Read the model definition and answer for the solid it produces. Units are mm, in the model's axes. Round coordinates to 2 decimals unless told otherwise and drop trailing zeros. Loops run counter-clockwise (first coordinate to the right, second up) from the corner with the lowest first, then second, coordinate; pieces in that order, holes last. Notation, with made-up numbers: M 61.5,75 L 69.5,75 A21 cw 69.5,108 Z; hole C 55,34 d4. An arc over 180 degrees is marked long. Write each question's results on one line, items separated by ' | '.
```python
from build123d import *

# Parameters (mm, degrees)
CYLINDER001_R     = 1.65
CYLINDER001_DEPTH = 3
CYLINDER_R        = 3.5
CYLINDER_DEPTH    = 3
CHAMFER001_SIZE   = 0.4


with BuildPart() as cylinder001:
    # Cylinder001 → Cylinder001 (new body)
    with BuildSketch(Plane.XY):
        Circle(CYLINDER001_R)
    extrude(amount=CYLINDER001_DEPTH)


with BuildPart() as chamfer001:
    # Cylinder → Cylinder (new body)
    with BuildSketch(Plane.XY):
        Circle(CYLINDER_R)
    extrude(amount=CYLINDER_DEPTH)

    # Cut: cut Cylinder001
    add(cylinder001.part, mode=Mode.SUBTRACT)

    # Chamfer001
    chamfer001_edges = [chamfer001.edges().sort_by_distance(p)[0] for p in [
        (-3.5, 0, 0),
        (-1.65, 0, 0),
    ]]
    chamfer(chamfer001_edges, length=CHAMFER001_SIZE)


solid = chamfer001.part
```
1. Find section C-C, the plane z = 1.3. Give the vertices of the cut face in (x, y).
Completed:
outline: C 0,0 d7; hole C 0,0 d3.3
2. Determine the mould class of faces 1 (the face through (1, -2, 3)), 2 (the face through (-1.216, 1.115, 1.682)), 3 (the face through (3.233, -1.341, 1.682)) for opening direction Y: released by +Y, released by -Y, zero draft, split by the parting line, or undercut.
Completed:
face 1: zero draft | face 2: undercut | face 3: split by the parting line
3. Find the intervals of material crossed by L1, parallel to Y at x = 0, z = 1.9; L2, parallel to X at y = 0.5, z = 0.65; L3, parallel to X at y = 1, z = 2.6, in increasing order.
Completed:
L1: y = -3.5 to -1.65, 1.65 to 3.5 | L2: x = -3.46 to -1.57, 1.57 to 3.46 | L3: x = -3.35 to -1.31, 1.31 to 3.35
4. Find section A-A, the plane y = 0. Give the vertices of the cut face in (x, z), then the cut area to 3 significant figures.
Completed:
outline: M -3.5,0.4 L -3.1,0 L -2.05,0 L -1.65,0.4 L -1.65,3 L -3.5,3 Z; M 1.65,0.4 L 2.05,0 L 3.1,0 L 3.5,0.4 L 3.5,3 L 1.65,3 Z | area: 10.8 mm2
